```python
from build123d import *

# Parameters (mm, degrees)
SKETCH1_R                     = 7.9375
BOSS_EXTRUDE1_DEPTH           = 6.35
SKETCH2_R                     = 16.4211
BOSS_EXTRUDE3_DEPTH           = 6.35
BOSS_EXTRUDE3_DEPTH_BACK      = 3.175
F_6_CLEARANCE_HOLE1_D         = 4.3053
F_6_CLEARANCE_HOLE1_DEPTH     = 9.525
F_6_PLASTIC_INSERT_AT_2_COUNT = 2
F_6_PLASTIC_INSERT_AT_2_PITCH = 46.355
BOSS_EXTRUDE4_REACH           = 14.7
SKETCH22_R                    = 16.4211
SKETCH22_R_2                  = 7.9375
CUT_EXTRUDE1_START            = -6.23
CUT_EXTRUDE1_DEPTH            = 6.23
SKETCH24_R                    = 1.5875
CUT_EXTRUDE2_DEPTH            = 13.7
HOLE1_AT_2_COUNT              = 2
HOLE1_AT_2_PITCH              = 27
F_0_CLEARANCE_HOLE1_D         = 1.8542


with BuildPart() as part:
    # Sketch1 → Boss-Extrude1 (new body)
    with BuildSketch(Plane.XY):
        with BuildLine():
            ThreePointArc((16.170566439, -2.8575), (16.4211, 0), (16.170566439, 2.8575))
            ThreePointArc((16.170566439, 2.8575), (0, 16.4211), (-16.170566439, 2.8575))
            ThreePointArc((-16.170566439, 2.8575), (-16.4211, 0), (-16.170566439, -2.8575))
            ThreePointArc((-16.170566439, -2.8575), (0, -16.4211), (16.170566439, -2.8575))
        make_face()
        Circle(SKETCH1_R, mode=Mode.SUBTRACT)
    extrude(amount=BOSS_EXTRUDE1_DEPTH)

    # Sketch2 → Boss-Extrude3 (add, two sides)
    with BuildSketch(Plane.XY.offset(6.35)) as boss_extrude3_sk:
        with BuildLine():
            Line((23.1775, 4.1275), (23.138323054, 4.1275))
            ThreePointArc((23.138323054, 4.1275), (19.696705066, 5.14104372), (17.35374229, 7.858125))
            ThreePointArc((17.35374229, 7.858125), (0, 19.05), (-17.35374229, 7.858125))
            ThreePointArc((-17.35374229, 7.858125), (-19.696705066, 5.14104372), (-23.138323054, 4.1275))
            Line((-23.138323054, 4.1275), (-23.1775, 4.1275))
            ThreePointArc((-23.1775, 4.1275), (-27.305, 0), (-23.1775, -4.1275))
            Line((-23.1775, -4.1275), (-23.138323054, -4.1275))
            ThreePointArc((-23.138323054, -4.1275), (-19.696705066, -5.14104372), (-17.35374229, -7.858125))
            ThreePointArc((-17.35374229, -7.858125), (0, -19.05), (17.35374229, -7.858125))
            ThreePointArc((17.35374229, -7.858125), (19.696705066, -5.14104372), (23.138323054, -4.1275))
            Line((23.138323054, -4.1275), (23.1775, -4.1275))
            ThreePointArc((23.1775, -4.1275), (27.305, 0), (23.1775, 4.1275))
        make_face()
        Circle(SKETCH2_R, mode=Mode.SUBTRACT)
    extrude(amount=BOSS_EXTRUDE3_DEPTH)
    extrude(boss_extrude3_sk.sketch, amount=-BOSS_EXTRUDE3_DEPTH_BACK)

    # #6 Clearance Hole1
    with Locations(Plane(origin=(-22.699598292, 0.104385938, 3.175), x_dir=(-1, 0, 0), z_dir=(0, 0, -1))):
        with Locations((-45.877098292, -0.104385938), (0.477901708, -0.104385938)):
            Hole(F_6_CLEARANCE_HOLE1_D / 2, depth=F_6_CLEARANCE_HOLE1_DEPTH)

    # Sketch5 → #6 Plastic Insert (revolve, cut)
    with BuildSketch(Plane(origin=(23.1775, 0, 3.175), x_dir=(0, 1, 0), z_dir=(1, 0, 0))):
        Polygon((0, 0), (0, 3.81), (2.5273, 3.81), (2.6543, 0), align=None)
    f_6_plastic_insert = revolve(axis=Axis((23.1775, 0, 113.175), (0, 0, -1)), mode=Mode.SUBTRACT)

    # #6 Plastic Insert at 2: #6 Plastic Insert ×2
    with Locations(*[(-i * F_6_PLASTIC_INSERT_AT_2_PITCH, 0, 0) for i in range(1, F_6_PLASTIC_INSERT_AT_2_COUNT)]):
        add(f_6_plastic_insert, mode=Mode.SUBTRACT)

    # Sketch22 → Boss-Extrude4 (add, up to next)
    with BuildSketch(Plane.XY.offset(12.7), mode=Mode.PRIVATE) as boss_extrude4_sk1:
        Circle(SKETCH22_R)
        Circle(SKETCH22_R_2, mode=Mode.SUBTRACT)
    boss_extrude4_tool1 = extrude(boss_extrude4_sk1.sketch, amount=-BOSS_EXTRUDE4_REACH, mode=Mode.PRIVATE) - part.part
    add(boss_extrude4_tool1.solids().sort_by_distance((-15.956641, 0, 12.7))[0])

    # Sketch23 → Cut-Extrude1 (cut)
    with BuildSketch(Plane.XY.offset(12.7).offset(CUT_EXTRUDE1_START)):
        with BuildLine():
            Line((-4.060251152, 10.629391126), (-10.629391126, 4.060251152))
            ThreePointArc((-10.629391126, 4.060251152), (-12.41058312, -4.506273431), (-9.348763248, -12.702812177))
            ThreePointArc((-9.348763248, -12.702812177), (-8.44083665, -15.052079048), (-6.091569778, -15.960005646))
            ThreePointArc((-6.091569778, -15.960005646), (14.451038284, -14.451038284), (15.960005646, 6.091569778))
            ThreePointArc((15.960005646, 6.091569778), (15.052079048, 8.44083665), (12.702812177, 9.348763248))
            ThreePointArc((12.702812177, 9.348763248), (4.506273431, 12.41058312), (-4.060251152, 10.629391126))
        make_face()
    extrude(amount=CUT_EXTRUDE1_DEPTH, mode=Mode.SUBTRACT)

    # Sketch24 → Cut-Extrude2 (cut, through all)
    with BuildSketch(Plane(origin=(0, 0, 0), x_dir=(-1, 0, 0), z_dir=(0, 0, -1))):
        with Locations((-7.548261886, -7.548261886)):
            Circle(SKETCH24_R)
    extrude(amount=-CUT_EXTRUDE2_DEPTH, mode=Mode.SUBTRACT)

    # Sketch26 → Hole1 (revolve, cut)
    with BuildSketch(Plane(origin=(-6.240320347, -12.851562745, 6.47), x_dir=(0, -1, 0), z_dir=(1, 0, 0))):
        Polygon((0, 0), (0, 2.921), (1.4986, 2.921), (1.6383, 0), align=None)
    hole1 = revolve(axis=Axis((-6.240320347, -12.851562745, -103.53), (0, 0, 1)), mode=Mode.SUBTRACT)

    # Hole1 at 2: Hole1 ×2
    with Locations(*[Vector(0.707106781, 0.707106781, 0) * (i * HOLE1_AT_2_PITCH) for i in range(1, HOLE1_AT_2_COUNT)]):
        add(hole1, mode=Mode.SUBTRACT)

    # #0 Clearance Hole1 (through all)
    with Locations(Plane.XY.offset(6.47)):
        with Locations((-6.240320347, -12.851562745), (12.851562745, 6.240320347)):
            Hole(F_0_CLEARANCE_HOLE1_D / 2)


solid = part.part
```
Source: CAD feature listing. Evaluate the final solid. Frame: model axes, mm. A direction names the side the tool comes from. Give positions to 0.01 mm unless a question says otherwise; leave off trailing zeros. Loops run counter-clockwise (first coordinate to the right, second up) from the corner with the lowest first, then second, coordinate; pieces in that order, holes last. Notation, with made-up numbers: (7.25, 2.5) - (47.25, 2.5) arc R14 cw to (47.25, 27.5) - close; hole circle Ø4 at (38, 34). An arc over 180 degrees is marked (long way). Use CSV: the item, a comma, the result in double quotes. Start each with the question number.
1. Ray query, L1, parallel to Y at x = 0, z = 4; L2, parallel to Y at x = 0, z = 1.75; L3, parallel to X at y = -1, z = 8.5. Return the intervals inside material, ascending.
2. Section A-A (z = 10.75). Count the separate pieces of the cut face and the enclosed holes in it, then the cut area to 3 significant figures.
3. Draft query along Y for faces 4 (the cylindrical face through (0.306, 19.048, 8.004)), 5 (the cylindrical face through (27.304, -0.091, 8.004)), 6 (the flat face through (12, 7, 3.549)). Return one class per face: +Y half, -Y half, draft (parallel to the pull), parting line (faces both ways), or undercut.
4. Section D-D (y = -10.5). Output: boundary loops of the cut face in (x, z) (3 decimals).
5. Pin query (flat end, axial travel): pin 1 (0.9 mm diameter, centred on x = 13.5, y = 6, fed in from +Z); pin 2 (0.9 mm diameter, centred on x = -6.5, y = -13, fed in from +Z); pin 3 (1.5 mm diameter, centred on x = 5, y = -11, fed in from +Z); pin 4 (3 mm diameter, centred on x = -15, z = 9.5, fed in from +Y). Return the tip coordinate at first contact, or that it passes through.
6. Reachability of faces 1 (the cylindrical face through (4.63, 12.4, 9.54)), 2 (the cylindrical face through (-25.33, 0.09, 9.88)), 3 (the flat face through (-22, -2, 6.985)) from +Z, -Z, +X, -X, +Y, -Y: full face, straight path, thin tool, end or side. Return the list, or none.
Response:
1,L1,"-19.05 to -7.94, 7.94 to 19.05"
1,L2,"-16.42 to -7.94, 7.94 to 16.42"
1,L3,"-27.18 to -25.08, -21.27 to -12.29, 18.9 to 21.27, 25.08 to 27.18"
2,separate pieces,"1"
2,enclosed holes,"2"
2,area,"490 mm²"
3,face 4,"+Y half"
3,face 5,"parting line"
3,face 6,"undercut"
4,outline,"(-15.895, 3.175) - (-12.625, 3.175) - (-12.625, 0) - (12.625, 0) - (12.625, 3.175) - (15.895, 3.175) - (15.895, 6.47) - (-10.719, 6.47) - (-10.719, 12.7) - (-15.895, 12.7) - close"
5,pin 1,"z = 3.55"
5,pin 2,"through"
5,pin 3,"z = 6.47"
5,pin 4,"y = 13.44"
6,face 1,"+Z"
6,face 2,"+Z, -Z"
6,face 3,"-Z"
